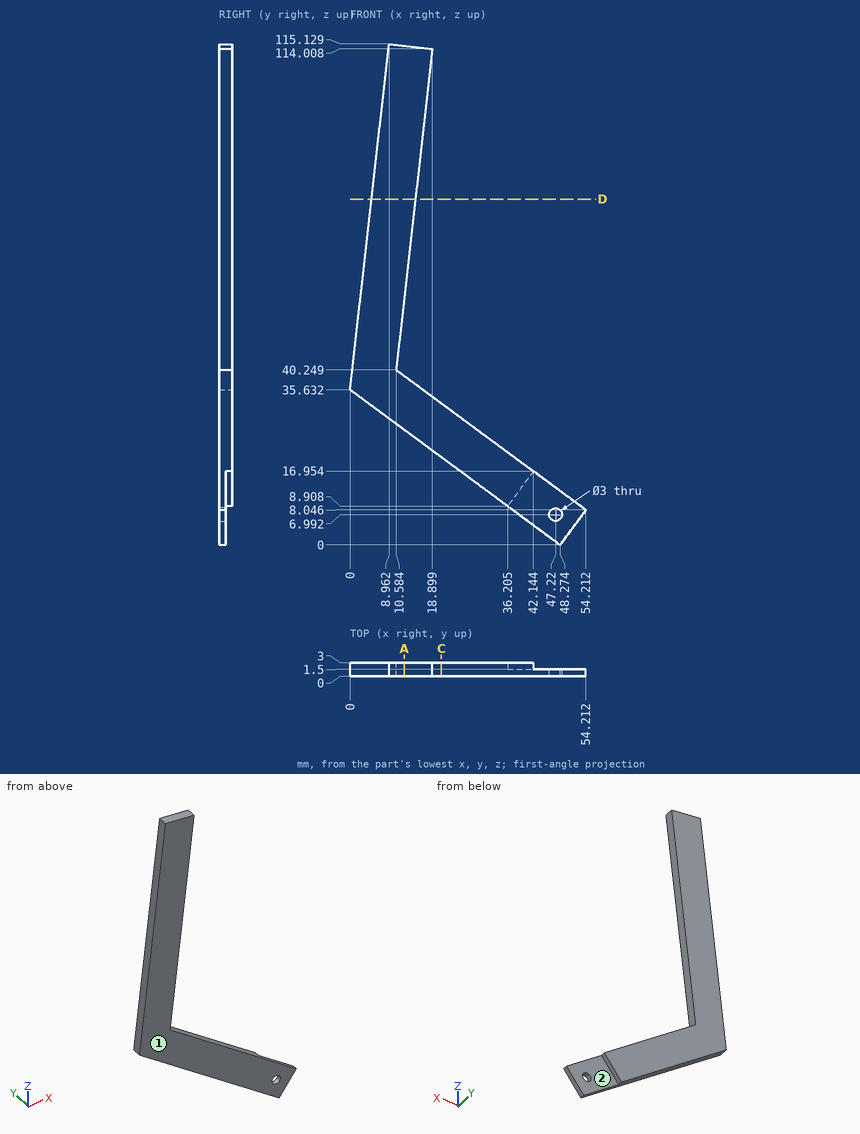
Here's the drawing with two shaded views (mm, measured from the low corner). I have some questions. A direction names the side the tool comes from. Coordinates: 2 decimals unless noted, no trailing zeros. Order: outer loops, then holes, each group sorted by start corner. A loop starts at its lowest first (then second) coordinate and runs counter-clockwise, first axis right, second up. Notation, with made-up numbers: (-11, -13) - (-6, -13) arc R12 ccw to (-6, -5) - close; hole circle Ø6 at (-14.5, -5). An arc over 180 degrees is marked (long way). Answer in a Markdown table with one row per item.
1. If I drill on line 1 along Z through (x, y) = (10, 1.1); line 2 along X through (y, z) = (0.15, 42.5) (1 decimal); line 3 along X through (y, z) = (1.6, 19) (1 decimal), over which ranges is the centre line in solid material (lowest first)?
Reply:
| item | result |
|---|---|
| line 1 | z = 28.25 to 115.01 |
| line 2 | x = 0.8 to 10.8 |
| line 3 | x = 22.5 to 39.4 |
2. Suppose I cut it at A-A (x = 12.5). Please give me the cut outline in (y, z) (1 decimal), and give its area (3 significant figures).
Reply:
| item | result |
|---|---|
| outline | (0, 26.4) - (3, 26.4) - (3, 38.8) - (0, 38.8) - close; (0, 57.2) - (3, 57.2) - (3, 114.7) - (0, 114.7) - close |
| area | 210 mm^2 |
3. For pin 1 (1.8 mm diameter, centred on x = 47.22, z = 6.99, fed in from +Y); pin 2 (1.5 mm diameter, centred on x = 41, y = 2, fed in from -Z) (1 decimal); pin 3 (1 mm diameter, centred on y = 2.5, z = 93.5, fed in from -X); pin 4 (1 mm diameter, centred on x = 16, y = 2, fed in from +Z), each with a flat end and sliding along its axis, tell me the tip position at first contact or that it passes through.
Reply:
| item | result |
|---|---|
| pin 1 | passes through |
| pin 2 | stops at z = 5 |
| pin 3 | stops at x = 6.47 |
| pin 4 | stops at z = 114.39 |
4. Suppose I cut it at C-C (x = 21). Please give me the cut outline in (y, z).
Reply:
| item | result |
|---|---|
| outline | (0, 20.13) - (3, 20.13) - (3, 32.56) - (0, 32.56) - close |
5. Suppose I cut it at D-D (z = 79.5). Please give me the cut outline in (x, y) (1 decimal), and give its area (3 significant figures).
Reply:
| item | result |
|---|---|
| outline | (4.9, 0) - (15, 0) - (15, 3) - (4.9, 3) - close |
| area | 30.2 mm^2 |
6. For the marked faces 1 and 2, which set-ups out of +Z, -Z, +X, -X, +Y, -Y let a thin tool reach every point of the face, with its end or its side?
Reply:
| item | result |
|---|---|
| face 1 | +Z, -Z, +X, -X, -Y |
| face 2 | -Z, +X, +Y |
